from build123d import *

# Parameters (mm, degrees)
SKETCH1_W            = 30
SKETCH1_H            = 103
BOSS_EXTRUDE1_DEPTH  = 5
SKETCH2_W            = 12
SKETCH2_H            = 3
SKETCH2_W_2          = 20
SKETCH2_H_2          = 82
CUT_EXTRUDE1_DEPTH   = 5
SKETCH3_W            = 5
SKETCH3_H            = 10
SKETCH3_H_2          = 5
BOSS_EXTRUDE2_DEPTH  = 55
SKETCH8_W            = 30
SKETCH8_H            = 103
BOSS_EXTRUDE6_DEPTH  = 5
SKETCH10_W           = 20
SKETCH10_H           = 82
SKETCH10_W_2         = 12
SKETCH10_H_2         = 3
CUT_EXTRUDE2_DEPTH   = 5
SKETCH22_W           = 5
SKETCH22_H           = 10
BOSS_EXTRUDE7_DEPTH  = 35
SKETCH23_W           = 30
SKETCH23_H           = 10
BOSS_EXTRUDE8_DEPTH  = 5
SKETCH25_W           = 5
SKETCH25_H           = 10
BOSS_EXTRUDE9_DEPTH  = 35
SKETCH26_W           = 30
SKETCH26_H           = 10
BOSS_EXTRUDE10_DEPTH = 5
SKETCH28_W           = 3
SKETCH28_H           = 10
CUT_EXTRUDE4_DEPTH   = 34


with BuildPart() as part:
    # Sketch1 → Boss-Extrude1 (new body)
    with BuildSketch(Plane(origin=(0, 0, 0), x_dir=(1, 0, 0), z_dir=(0, 1, 0))):
        with Locations((-3.526120729, 0.1485026)):
            Rectangle(SKETCH1_W, SKETCH1_H)
    extrude(amount=BOSS_EXTRUDE1_DEPTH)

    # Sketch2 → Cut-Extrude1 (cut)
    with BuildSketch(Plane(origin=(0, 5, 0), x_dir=(1, 0, 0), z_dir=(0, 1, 0))):
        with Locations((-3.526120729, 45.1485026)):
            Rectangle(SKETCH2_W, SKETCH2_H)
        with Locations((-3.526120729, -10.3514974)):
            Rectangle(SKETCH2_W_2, SKETCH2_H_2)
    extrude(amount=-CUT_EXTRUDE1_DEPTH, mode=Mode.SUBTRACT)

    # Sketch3 → Boss-Extrude2 (add)
    with BuildSketch(Plane.XZ):
        with Locations((-16.026120729, 46.3514974)):
            Rectangle(SKETCH3_W, SKETCH3_H)
        with Locations((-16.026120729, -33.1485026)):
            Rectangle(SKETCH3_W, SKETCH3_H_2)
        with Locations((8.973879271, 46.3514974)):
            Rectangle(SKETCH3_W, SKETCH3_H)
        with Locations((8.973879271, -33.1485026)):
            Rectangle(SKETCH3_W, SKETCH3_H_2)
    extrude(amount=BOSS_EXTRUDE2_DEPTH)

    # Sketch8 → Boss-Extrude6 (add)
    with BuildSketch(Plane(origin=(0, -55, 0), x_dir=(-1, 0, 0), z_dir=(0, -1, 0))):
        with Locations((3.526120729, 0.1485026)):
            Rectangle(SKETCH8_W, SKETCH8_H)
    extrude(amount=BOSS_EXTRUDE6_DEPTH)

    # Sketch10 → Cut-Extrude2 (cut)
    with BuildSketch(Plane.XZ.offset(60)):
        with Locations((-3.526120729, 10.3514974)):
            Rectangle(SKETCH10_W, SKETCH10_H)
        with Locations((-3.526120729, -45.1485026)):
            Rectangle(SKETCH10_W_2, SKETCH10_H_2)
    extrude(amount=-CUT_EXTRUDE2_DEPTH, mode=Mode.SUBTRACT)

    # Sketch22 → Boss-Extrude7 (add)
    with BuildSketch(Plane(origin=(0, 5, 0), x_dir=(1, 0, 0), z_dir=(0, 1, 0))):
        with Locations((-16.026120729, -46.3514974)):
            Rectangle(SKETCH22_W, SKETCH22_H)
        with Locations((8.973879271, -46.3514974)):
            Rectangle(SKETCH22_W, SKETCH22_H)
    extrude(amount=BOSS_EXTRUDE7_DEPTH)

    # Sketch23 → Boss-Extrude8 (add)
    with BuildSketch(Plane(origin=(0, 40, 0), x_dir=(1, 0, 0), z_dir=(0, 1, 0))):
        with Locations((-3.526120729, -46.3514974)):
            Rectangle(SKETCH23_W, SKETCH23_H)
    extrude(amount=BOSS_EXTRUDE8_DEPTH)

    # Sketch25 → Boss-Extrude9 (add)
    with BuildSketch(Plane(origin=(0, -60, 0), x_dir=(-1, 0, 0), z_dir=(0, -1, 0))):
        with Locations((16.026120729, -46.3514974)):
            Rectangle(SKETCH25_W, SKETCH25_H)
        with Locations((-8.973879271, -46.3514974)):
            Rectangle(SKETCH25_W, SKETCH25_H)
    extrude(amount=BOSS_EXTRUDE9_DEPTH)

    # Sketch26 → Boss-Extrude10 (add)
    with BuildSketch(Plane.XZ.offset(95)):
        with Locations((-3.526120729, 46.3514974)):
            Rectangle(SKETCH26_W, SKETCH26_H)
    extrude(amount=BOSS_EXTRUDE10_DEPTH)

    # Sketch28 → Cut-Extrude4 (cut)
    with BuildSketch(Plane(origin=(11.473879271, 0, 0), x_dir=(0, 0, -1), z_dir=(1, 0, 0))):
        with Locations((-46.8514974, 10)):
            Rectangle(SKETCH28_W, SKETCH28_H)
        with Locations((-46.8514974, -65)):
            Rectangle(SKETCH28_W, SKETCH28_H)
    extrude(amount=-CUT_EXTRUDE4_DEPTH, mode=Mode.SUBTRACT)


solid = part.part
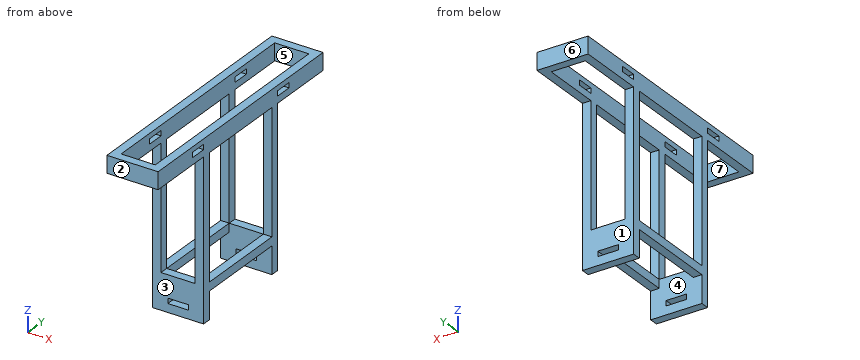
The model under review builds one solid part; all positions refer to its coordinate system, in mm. Face numbers are marked on the shaded views. A direction names the side the tool comes from. Give positions to 0.01 mm unless a question says otherwise; leave off trailing zeros. Order: outer loops, then holes, each group sorted by start corner. A loop starts at its lowest first (then second) coordinate and runs counter-clockwise, first axis right, second up. Notation, with made-up numbers: M 77.5,-7.75 L 101.5,-7.75 A28 cw 101.5,22.25 Z; hole C 68.5,34 d2. An arc over 180 degrees is marked long. Answer in a Markdown table with one row per item. Add a question column.
1. For pin 1 Ø9 at (x, z) = (-10, 5.5) entering from -Y; pin 2 Ø12 at (x, z) = (-10.5, 30.5) entering from +Y; pin 3 Ø4 at (x, y) = (8, -63.5) entering from -Z, all flat-tipped, find the tip position at first contact; note any pin that passes through.
2. Machinability: for the marked faces 1, 2, 3 and 4, which of the approach directions +Z, -Z, +X, -X, +Y, -Y give a long, thin tool a straight path to every point of the face, cutting with its end or side? Answer none if there is none.
3. Add section A-A on y = -74.5. State the section outline as (x, z) points, plus the area to 3 significant figures.
4. Add section C-C on z = -12. State the section outline as (x, y) points.
5. Mouldability with a two-part tool opening along X and no side actions: class the marked faces 5, 6 and 7 as released by +X, released by -X, zero draft, split by the parting line, or undercut.
6. To check wall thickness, follow line 1 along Z through (x, y) = (7.25, -16); line 2 along Y through (x, z) = (5, -31.5); line 3 along X through (y, z) = (-57.5, 9). State the ranges of each line that lie inside material, in increasing order.
7. Add section D-D on x = -4.5. State the section outline as (y, z) points, plus the area to 3 significant figures.
8. Add section B-B on x = 9.25. State the section outline as (y, z) points, plus the area to 4 significant figures.
The answers:
| question | item | result |
|---|---|---|
| 1 | pin 1 | y = -60 |
| 1 | pin 2 | y = 5 |
| 1 | pin 3 | z = 41.35 |
| 2 | face 1 | -Z, +X, -X, +Y |
| 2 | face 2 | +Z, -Z, +X, -X, -Y |
| 2 | face 3 | -Z, +X, -X, -Y |
| 2 | face 4 | -Z |
| 3 | outline | M -18.53,41.35 L -13.53,41.35 L -13.53,51.35 L -18.53,51.35 Z; M 6.47,41.35 L 11.47,41.35 L 11.47,51.35 L 6.47,51.35 Z |
| 3 | area | 100 mm2 |
| 4 | outline | M -18.53,-60 L -13.53,-60 L -13.53,-55 L -18.53,-55 Z; M -18.53,0 L -13.53,0 L -13.53,5 L -18.53,5 Z; M 6.47,-60 L 11.47,-60 L 11.47,-55 L 6.47,-55 Z; M 6.47,0 L 11.47,0 L 11.47,5 L 6.47,5 Z |
| 5 | face 5 | undercut |
| 5 | face 6 | zero draft |
| 5 | face 7 | undercut |
| 6 | line 1 | -35.65 to -30.65, 41.35 to 51.35 |
| 6 | line 2 | -60 to -55, 0 to 5 |
| 6 | line 3 | -18.53 to -13.53, 6.47 to 11.47 |
| 7 | outline | M -100,41.35 L -95,41.35 L -95,51.35 L -100,51.35 Z; M -60,-51.65 L -55,-51.65 L -55,-46.65 L -60,-46.65 Z; M -60,-43.65 L -55,-43.65 L -55,-30.65 L -60,-30.65 Z; M 0,-51.65 L 5,-51.65 L 5,-46.65 L 0,-46.65 Z; M 0,-43.65 L 5,-43.65 L 5,-30.65 L 0,-30.65 Z; M 40,41.35 L 45,41.35 L 45,51.35 L 40,51.35 Z |
| 7 | area | 280 mm2 |
| 8 | outline | M -100,41.35 L -60,41.35 L -60,-51.65 L -55,-51.65 L -55,-35.65 L 0,-35.65 L 0,-51.65 L 5,-51.65 L 5,41.35 L 45,41.35 L 45,51.35 L -100,51.35 Z; hole M -70,45.35 L -60,45.35 L -60,48.35 L -70,48.35 Z; hole M -55,-30.65 L 0,-30.65 L 0,41.35 L -55,41.35 Z; hole M 5,45.35 L 15,45.35 L 15,48.35 L 5,48.35 Z |
| 8 | area | 2,595 mm2 |
